Part print with two shaded views. Sizes in mm from the minimum x, y, z corner. A direction names the side the tool comes from. Round coordinates to 2 decimals unless told otherwise and drop trailing zeros. Order: outer loops, then holes, each group sorted by start corner. A loop starts at its lowest first (then second) coordinate and runs counter-clockwise, first axis right, second up. Notation, with made-up numbers: (-10, 7.25) -> (47, 7.25) arc R11 ccw to (47, 15.25) -> close; hole circle Ø9 at (-15.5, 7). An arc over 180 degrees is marked (long way). Put each result on its own line as item: value. Start each with the question number.
Q1. Pull direction X, two halves, no side cores. Call the marked faces 3, 4 and 5: released by +X, released by -X, zero draft, split by the parting line, or undercut.
Q2. 3-axis set-ups, long thin cutter, end or side, ignore diameter. For the marked faces 1 and 2: which of +Z, -Z, +X, -X, +Y, -Y reach the whole face in a straight line?
Q3. Cut at B-B, the plane z = 8. List the corners of the cut face in (x, y), and give its area (3 significant figures).
Q4. Flat gauge pin, fed straight in: P1, Ø3.5, axis at x = 67, y = 58, coming from the +Z side. Where does the tip first touch, or does it go through?
Q5. Probe L1, parallel to X at y = 42.5, z = 5; L2, parallel to Y at x = 64, z = 18.5; L3, parallel to Y at x = 7, z = 48.5 (1 decimal). List the from-to ranges inside material, lowest first.
Q6. Cut at D-D, the plane z = 59.5. List the corners of the cut face in (x, y) (1 decimal), and give its area (3 significant figures).
Q7. Cut at A-A, the plane y = 36.5. List the corners of the cut face in (x, z).
Q8. Cut at C-C, the plane x = 16. List the corners of the cut face in (y, z), and give its area (3 significant figures).
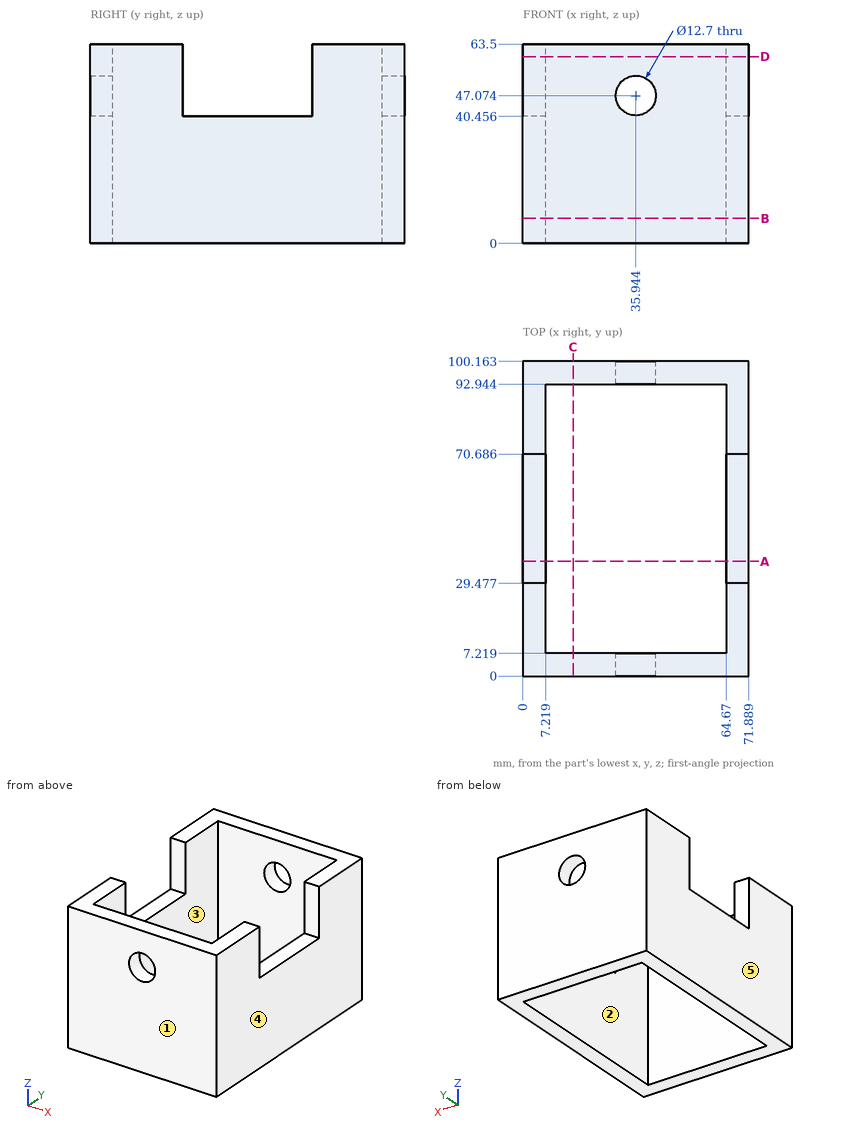
Ans:
1. face 3: undercut
1. face 4: released by +X
1. face 5: released by -X
2. face 1: +Z, -Z, +X, -X, -Y
2. face 2: +Z, -Z
3. outline: (0, 0) -> (71.89, 0) -> (71.89, 100.16) -> (0, 100.16) -> close; hole (7.22, 7.22) -> (64.67, 7.22) -> (64.67, 92.94) -> (7.22, 92.94) -> close
3. area: 2,280 mm^2
4. P1: stops at z = 40.46
5. L1: x = 0 to 7.22, 64.67 to 71.89
5. L2: y = 0 to 7.22, 92.94 to 100.16
5. L3: y = 0 to 29.5, 70.7 to 100.2
6. outline: (0, 0) -> (71.9, 0) -> (71.9, 29.5) -> (64.7, 29.5) -> (64.7, 7.2) -> (7.2, 7.2) -> (7.2, 29.5) -> (0, 29.5) -> close; (0, 70.7) -> (7.2, 70.7) -> (7.2, 92.9) -> (64.7, 92.9) -> (64.7, 70.7) -> (71.9, 70.7) -> (71.9, 100.2) -> (0, 100.2) -> close
6. area: 1,680 mm^2
7. outline: (0, 0) -> (7.22, 0) -> (7.22, 40.46) -> (0, 40.46) -> close; (64.67, 0) -> (71.89, 0) -> (71.89, 40.46) -> (64.67, 40.46) -> close
8. outline: (0, 0) -> (7.22, 0) -> (7.22, 63.5) -> (0, 63.5) -> close; (92.94, 0) -> (100.16, 0) -> (100.16, 63.5) -> (92.94, 63.5) -> close
8. area: 917 mm^2
